The drawing under review shows one solid part. Ordinate dimensions are in mm from its lowest x, y, z. A direction names the side the tool comes from. Coordinates: 2 decimals unless noted, no trailing zeros. Write each loop counter-clockwise with the first axis right and the second up, starting at its lowest first coordinate (ties: lowest second). Pieces come first, ordered by that corner, then holes.
Q1. Mouldability with a two-part tool opening along Z and no side actions: class the marked faces 1, 2, 3 and 4 as pulls with the +Z half, pulls with the -Z half, needs draft (parallel to the pull), parting line crosses it, or undercut.
Q2. Take a section at D-D (x = 13). Give the boundary of the cut face in (y, z).
Q3. Machinability: for the marked faces 5 and 6, which of the approach directions +Z, -Z, +X, -X, +Y, -Y give a long, thin tool a straight path to every point of the face, cutting with its end or side? Answer none if there is none.
Q4. For probe 1 along Z at (x, y) = (12, 0.75); probe 2 along Z at (x, y) = (12, 4.5); probe 3 along X at (y, z) = (4.55, 6), list the stretches that pass through material, from the lowest coordinate up.
Q5. Take a section at A-A (z = 34). Give the boundary of the cut face in (x, y), and give its area (3 significant figures).
Q6. Take a section at B-B (x = 16.5). Give the boundary of the cut face in (y, z), and give its area (3 significant figures).
Q7. Insertion check: pin 1 (3 mm diameter, centred on x = 12, z = 6, fed in from -Y); pin 2 (3 mm diameter, centred on x = 12.5, z = 33.5, fed in from -Y). Each pin has a flat end and moves straight along its axis. Give the tip position at first contact, or say it passes through.
Q8. Take a section at C-C (y = 3.8). Give the boundary of the cut face in (x, z), and give its area (3 significant figures).
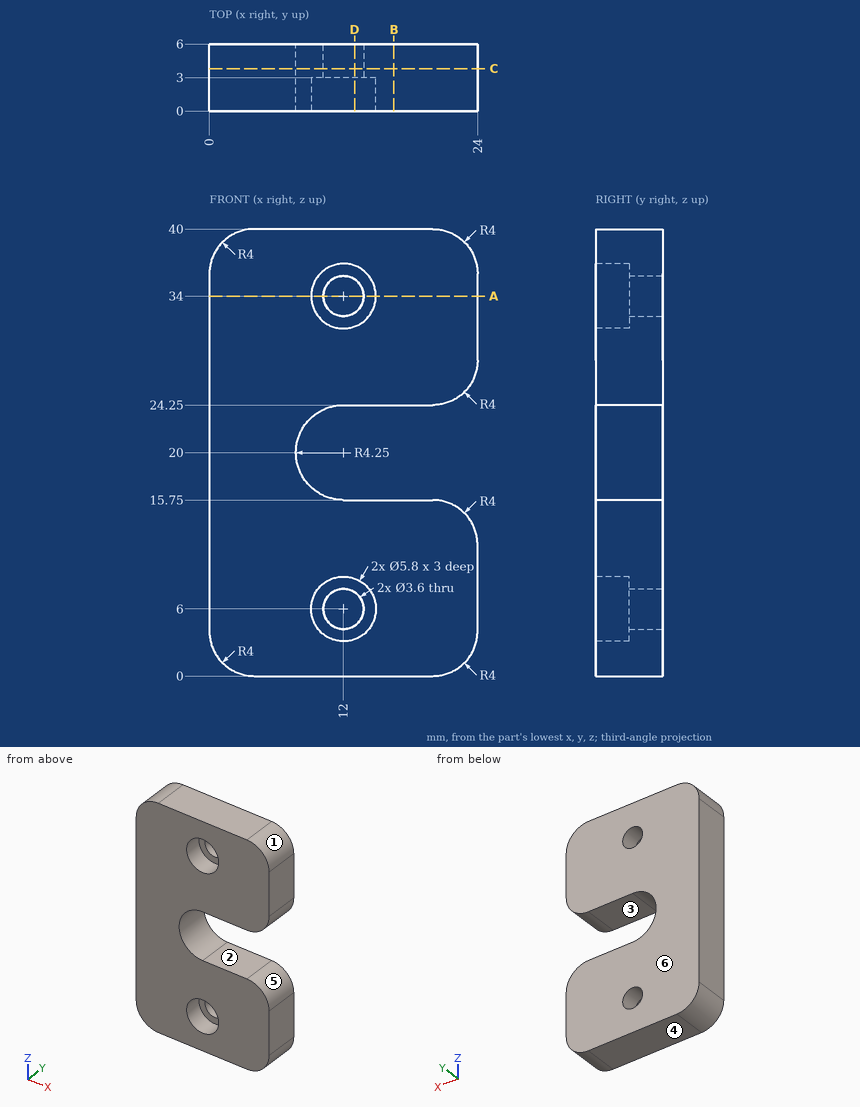
Response:
1. face 1: pulls with the +Z half
1. face 2: undercut
1. face 3: undercut
1. face 4: pulls with the -Z half
2. outline: (0, 0) - (6, 0) - (6, 4.5) - (3, 4.5) - (3, 3.28) - (0, 3.28) - close; (0, 8.72) - (3, 8.72) - (3, 7.5) - (6, 7.5) - (6, 15.75) - (0, 15.75) - close; (0, 24.25) - (6, 24.25) - (6, 32.5) - (3, 32.5) - (3, 31.28) - (0, 31.28) - close; (0, 36.72) - (3, 36.72) - (3, 35.5) - (6, 35.5) - (6, 40) - (0, 40) - close
3. face 5: +X, +Y, -Y
3. face 6: +Z, -Z, +X, -X, +Y
4. probe 1: z = 0 to 3.1, 8.9 to 15.75, 24.25 to 31.1, 36.9 to 40
4. probe 2: z = 0 to 4.2, 7.8 to 15.75, 24.25 to 32.2, 35.8 to 40
4. probe 3: x = 0 to 10.2, 13.8 to 24
5. outline: (0, 0) - (9.1, 0) - (9.1, 3) - (10.2, 3) - (10.2, 6) - (0, 6) - close; (13.8, 3) - (14.9, 3) - (14.9, 0) - (24, 0) - (24, 6) - (13.8, 6) - close
5. area: 116 mm2
6. outline: (0, 0) - (6, 0) - (6, 15.75) - (0, 15.75) - close; (0, 24.25) - (6, 24.25) - (6, 40) - (0, 40) - close
6. area: 189 mm2
7. pin 1: passes through
7. pin 2: stops at y = 3
8. outline: (0, 4) arc R4 ccw to (4, 0) - (20, 0) arc R4 ccw to (24, 4) - (24, 11.75) arc R4 ccw to (20, 15.75) - (12, 15.75) arc R4.25 cw to (12, 24.25) - (20, 24.25) arc R4 ccw to (24, 28.25) - (24, 36) arc R4 ccw to (20, 40) - (4, 40) arc R4 ccw to (0, 36) - close; hole circle Ø3.6 at (12, 6); hole circle Ø3.6 at (12, 34)
8. area: 789 mm2
